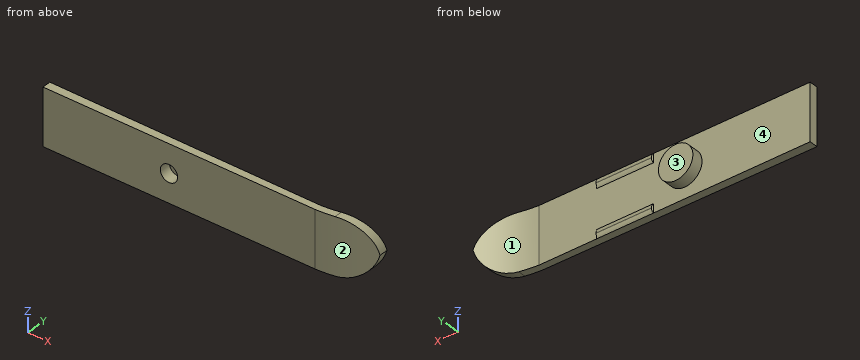
from build123d import *

# Parameters (mm, degrees)
SKATEBOARDBASE_DEPTH         = 7.9
CURVEDFRONT_R                = 5
SKETCH2_R                    = 2.4
STUD_DEPTH                   = 1.6
SKETCH3_W                    = 7.922196178
SKETCH3_H                    = 1.23692935
UPPERNOTCHES_DEPTH           = 0.2
UPPERNOTCHES_DRAFT           = 30
UPPERNOTCHES_PROFILE_2_DEPTH = 0.2
UPPERNOTCHES_PROFILE_2_DRAFT = 30
NOTCHFILLET_R                = 1
SKETCH4_R                    = 1.2
UNDERSTUDHOLE_DEPTH          = 1.6


with BuildPart() as part:
    # Sketch1 → SkateBoardBase (new body)
    with BuildSketch(Plane.XY):
        with BuildLine():
            Line((-20.371469293, 0.013768995), (17.388032716, 0.222549812))
            ThreePointArc((17.388032716, 0.222549812), (21.281619196, 0.833021385), (24.938309637, 2.303159558))
            Line((24.938309637, 2.303159558), (24.938309637, 3.514270646))
            ThreePointArc((24.938309637, 3.514270646), (21.290682244, 1.944239503), (17.388032716, 1.209726022))
            Line((17.388032716, 1.209726022), (-20.371469293, 1.209726022))
            Line((-20.371469293, 1.209726022), (-20.371469293, 0.013768995))
        make_face()
    extrude(amount=SKATEBOARDBASE_DEPTH)

    # CurvedFront
    # the kernel refuses this fillet: 5 mm, written as the material it takes off along each edge
    with BuildSketch(Plane(origin=(24.938309637, -10.196840442, 0), x_dir=(0, 0, 1), z_dir=(0, 1, 0))) as curvedfront_piece_1:
        with BuildLine():
            CenterArc((CURVEDFRONT_R, -CURVEDFRONT_R), CURVEDFRONT_R, 90, 90)
            Line((0, -CURVEDFRONT_R), (0, 0))
            Line((0, 0), (CURVEDFRONT_R, 0))
        make_face()
    extrude(amount=26.211111088, mode=Mode.SUBTRACT)
    with BuildSketch(Plane(origin=(24.938309637, -10.196840442, 7.9), x_dir=(0, 0, -1), z_dir=(0, 1, 0))) as curvedfront_piece_2:
        with BuildLine():
            CenterArc((CURVEDFRONT_R, CURVEDFRONT_R), CURVEDFRONT_R, 180, 90)
            Line((0, CURVEDFRONT_R), (0, 0))
            Line((0, 0), (CURVEDFRONT_R, 0))
        make_face()
    extrude(amount=26.211111088, mode=Mode.SUBTRACT)

    # Sketch2 → Stud (add)
    with BuildSketch(Plane(origin=(0, 1.209726022, 0), x_dir=(1, 0, 0), z_dir=(0, 1, 0))):
        with Locations(Location((-2.902006395, -3.95, 0), (0, 0, 90))):
            Circle(SKETCH2_R)
    extrude(amount=STUD_DEPTH)


with BuildPart() as uppernotches_tool:
    # Sketch3 → UpperNotches (with draft: the straight prism first)
    with BuildSketch(Plane(origin=(0, 1.209726022, 0), x_dir=(1, 0, 0), z_dir=(0, 1, 0))):
        with Locations((5.4387323, -0.618464675)):
            Rectangle(SKETCH3_W, SKETCH3_H)
    extrude(amount=UPPERNOTCHES_DEPTH)
    # UpperNotches: the draft: its side faces are tilted about the plane it starts from
    uppernotches_sides = [uppernotches_tool.faces().sort_by_distance(p)[0] for p in [
        (1.477634211, 1.309726022, 0.618464675),
        (5.4387323, 1.309726022, 1.23692935),
        (9.399830389, 1.309726022, 0.618464675),
        (5.4387323, 1.309726022, 0),
    ]]
    draft(uppernotches_sides, Plane(origin=(0, 1.209726022, 0), x_dir=(1, 0, 0), z_dir=(0, 1, 0)), UPPERNOTCHES_DRAFT)


with BuildPart() as part_1:
    add(part.part)

    # UpperNotches: add uppernotches_tool
    add(uppernotches_tool.part)


with BuildPart() as uppernotches_profile_2_tool:
    # Sketch3 → UpperNotches profile 2 (with draft: the straight prism first)
    with BuildSketch(Plane(origin=(0, 1.209726022, 0), x_dir=(1, 0, 0), z_dir=(0, 1, 0))):
        with Locations((5.4387323, -7.281535325)):
            Rectangle(SKETCH3_W, SKETCH3_H)
    extrude(amount=UPPERNOTCHES_PROFILE_2_DEPTH)
    # UpperNotches profile 2: the draft: its side faces are tilted about the plane it starts from
    uppernotches_profile_2_sides = [uppernotches_profile_2_tool.faces().sort_by_distance(p)[0] for p in [
        (5.4387323, 1.309726022, 6.66307065),
        (1.477634211, 1.309726022, 7.281535325),
        (5.4387323, 1.309726022, 7.9),
        (9.399830389, 1.309726022, 7.281535325),
    ]]
    draft(uppernotches_profile_2_sides, Plane(origin=(0, 1.209726022, 0), x_dir=(1, 0, 0), z_dir=(0, 1, 0)), UPPERNOTCHES_PROFILE_2_DRAFT)


with BuildPart() as part_2:
    add(part_1.part)

    # UpperNotches profile 2: add uppernotches_profile_2_tool
    add(uppernotches_profile_2_tool.part)

    # NotchFillet
    # the kernel refuses this fillet: 1 mm, written as the material it takes off along each edge
    with BuildSketch(Plane(origin=(0.381779399, 1.409726022, 1.121459296), x_dir=(0, -0.8660254037844376, 0.5000000000000017), z_dir=(1, 0, 0)), Plane(origin=(10.4956852, 1.409726022, 0.115470054), x_dir=(0, -0.8660254037844383, -0.5000000000000008), z_dir=(-1, 0, 0)), Plane(origin=(0.381779399, 1.409726022, 7.784529946), x_dir=(0, -0.8660254037844378, 0.5000000000000013), z_dir=(1, 0, 0)), Plane(origin=(10.4956852, 1.409726022, 6.778540704), x_dir=(0, -0.8660254037844378, -0.5000000000000013), z_dir=(-1, 0, 0))) as notchfillet_piece_1:
        with BuildLine():
            CenterArc((0.623760431, 0.919615242), NOTCHFILLET_R, 210, 36.869897646)
            Line((-0.242264973, 0.419615242), (-0.259585481, 0.409615242))
            Line((-0.259585481, 0.409615242), (-0.017320508, -0.01))
            Line((-0.017320508, -0.01), (0, -0.02))
            ThreePointArc((0, -0.02), (0.115470054, -0.02), (0.223083701, -0.018392305))
            Line((0.223083701, -0.018392305), (0.230940108, 0))
        make_face()
    extrude(amount=10.113905801, mode=Mode.SUBTRACT)

    # Sketch4 → UnderStudHole (cut)
    with BuildSketch(Plane(origin=(-0.000698914, 0.126403586, 0), x_dir=(-0.9999847141809186, -0.005529141389625959, 0), z_dir=(0.005529141389625959, -0.9999847141809186, 0))):
        with Locations(Location((2.895273289, -3.95, 0), (0, 0, 180))):
            Circle(SKETCH4_R)
    extrude(amount=-UNDERSTUDHOLE_DEPTH, mode=Mode.SUBTRACT)


solid = part_2.part
Geometry check sheet. Reference: the model listing, model coordinates, mm. Face numbers are marked on the shaded views. Round coordinates to 2 decimals unless told otherwise and drop trailing zeros. Order: outer loops, then holes, each group sorted by start corner. A loop starts at its lowest first (then second) coordinate and runs counter-clockwise, first axis right, second up. Notation, with made-up numbers: M 78,31.5 L 94,31.5 A14 cw 94,45.5 Z; hole C 8,53 d7. An arc over 180 degrees is marked long. Answer in a Markdown table with one row per item.
(1) Draft check along X on the marked faces 1, 2, 3 and 4. Enter one of: released by +X, released by -X, zero draft, split by the parting line, or undercut.
Responses:
| item | result |
|---|---|
| face 1 | undercut |
| face 2 | released by +X |
| face 3 | zero draft |
| face 4 | undercut |
(2) Sectioned sample at C-C, the plane z = 5.75. Record the cut outline in (x, y), and give its area (3 significant figures).
Responses:
| item | result |
|---|---|
| outline | M -20.37,0.01 L 17.39,0.22 A17.42 ccw 24.05,1.85 L 24.05,3.04 A18.05 cw 17.39,1.21 L -1.31,1.21 L -1.31,2.81 L -4.49,2.81 L -4.49,1.21 L -20.37,1.21 Z |
| area | 53.6 mm² |
(3) Sectioned sample at A-A, the plane z = 3.5. Record the cut outline in (x, y).
Responses:
| item | result |
|---|---|
| outline | M -20.37,0.01 L -4.01,0.1 L -4.02,1.7 L -1.79,1.72 L -1.78,0.12 L 17.39,0.22 A17.42 ccw 24.71,2.18 L 24.71,3.39 A18.05 cw 17.39,1.21 L -0.54,1.21 L -0.54,2.81 L -5.26,2.81 L -5.26,1.21 L -20.37,1.21 Z |
(4) Sectioned sample at B-B, the plane x = -1. Record the cut outline in (y, z), and give its area (3 significant figures).
Responses:
| item | result |
|---|---|
| outline | M 0.12,0 L 1.21,0 L 1.21,2.49 L 2.81,2.49 L 2.81,5.41 L 1.21,5.41 L 1.21,7.9 L 0.12,7.9 Z |
| area | 13.3 mm² |
(5) Scan lines: probe 1 along X at (y, z) = (2.55, 5.5); probe 2 along Z at (x, y) = (21, 1.15); probe 3 along Y at (x, z) = (9.5, 4.5). Record each from-to range of solid material in increasing order. Write a range as from..to.
Responses:
| item | result |
|---|---|
| probe 1 | x = -4.73..-1.07, 22.97..24.21 |
| probe 2 | z = 0.11..7.79 |
| probe 3 | y = 0.18..1.21 |
(6) Sectioned sample at D-D, the plane x = 13.5. Record the cut outline in (y, z).
Responses:
| item | result |
|---|---|
| outline | M 0.2,0 L 1.21,0 L 1.21,7.9 L 0.2,7.9 Z |
